Can you work these out from the model? Positions are in its coordinate system, mm. Face numbers are marked on the shaded views. A direction names the side the tool comes from. Give positions to 0.01 mm unless a question says otherwise; leave off trailing zeros. Order: outer loops, then holes, each group sorted by start corner. A loop starts at its lowest first (then second) coordinate and runs counter-clockwise, first axis right, second up. Notation, with made-up numbers: M -26.5,-15 L 9.5,-15 A21 cw 9.5,-1 Z; hole C -26.75,40 d6. An arc over 180 degrees is marked long. Answer as a JSON object with one key per item and string values.
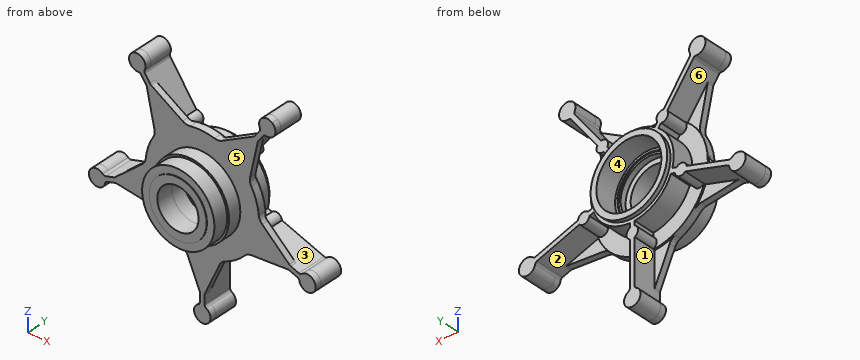
```python
from build123d import *
from build123d.topology import SkipClean

# Parameters (mm, degrees)
BOSS_EXTRUDE1_DEPTH     = 21
CIRPATTERN1_COUNT       = 5
SKETCH3_R               = 294.674158119
SKETCH3_R_2             = 133.5
CUT_EXTRUDE1_DEPTH      = 3.5
BOSS_EXTRUDE2_START     = 68
BOSS_EXTRUDE2_DEPTH     = 68
CIRPATTERN2_COUNT       = 5
SKETCH6_R               = 312.065811201
CUT_EXTRUDE3_DEPTH      = 15
SKETCH7_R               = 90
SKETCH7_R_2             = 71
BOSS_EXTRUDE3_DEPTH     = 9
SKETCH8_R               = 76.5
CUT_EXTRUDE4_DEPTH      = 50
SKETCH9_R               = 313.84536257
SKETCH9_R_2             = 94
CUT_EXTRUDE5_DEPTH      = 3
SKETCH10_R              = 106.760596323
SKETCH10_R_2            = 85
CUT_EXTRUDE6_DEPTH      = 34
SKETCH11_R              = 112.872926099
SKETCH11_R_2            = 89.5
CUT_EXTRUDE7_DEPTH      = 30
SKETCH12_R              = 67.5
SKETCH12_R_2            = 45
BOSS_EXTRUDE4_DEPTH     = 1
CUT_EXTRUDE8_DEPTH      = 412.038532061
CUT_EXTRUDE8_DEPTH_BACK = 412.038532061
SKETCH13_R              = 48.5


with BuildPart() as part:
    # Sketch1 → Revolve1 (revolve)
    with BuildSketch(Plane.XY, mode=Mode.PRIVATE) as revolve1_sk:
        with BuildLine():
            Line((89.84228169, 2.60989789), (97.5, 61))
            Line((97.5, 61), (133.5, 61))
            Line((133.5, 61), (133.5, 82))
            Line((133.5, 82), (97.5, 82))
            Line((97.5, 82), (97.5, 147))
            Line((97.5, 147), (71, 147))
            Line((71, 147), (71, 88))
            Line((71, 88), (66, 88))
            Line((66, 88), (66, 75))
            Line((66, 75), (54, 75))
            Line((54, 75), (51.505319297, 40.981626783))
            Line((51.505319297, 40.981626783), (50.883331755, 40.539778313))
            Line((50.883331755, 40.539778313), (48.5, 0))
            Line((48.5, 0), (86.867753099, 0))
            ThreePointArc((86.867753099, 0), (88.846350287, 0.744971582), (89.84228169, 2.60989789))
        make_face()
    revolve(revolve1_sk.sketch.rotate(Axis((0, 165, 0), (0, -1, 0)), 180), axis=Axis((0, 165, 0), (0, -1, 0)))

    # Sketch2 → Boss-Extrude1 (add)
    with BuildSketch(Plane(origin=(0, 82, 0), x_dir=(1, 0, 0), z_dir=(0, 1, 0))):
        with BuildLine():
            Line((-6.35450353, 213.067894216), (-40.878618186, 135.005909342))
            ThreePointArc((-40.878618186, 135.005909342), (-46.087052335, 127.41774711), (-53.688359463, 122.228515733))
            ThreePointArc((-53.688359463, 122.228515733), (0, 133.5), (53.688359463, 122.228515733))
            ThreePointArc((53.688359463, 122.228515733), (46.087052335, 127.41774711), (40.878618186, 135.005909342))
            Line((40.878618186, 135.005909342), (6.35450353, 213.067894216))
            ThreePointArc((6.35450353, 213.067894216), (5.71595777, 215.045623904), (5.5, 217.112630835))
            Line((5.5, 217.112630835), (5.5, 236.859260412))
            ThreePointArc((5.5, 236.859260412), (6.48800918, 240.444782185), (9.173133251, 243.018152978))
            ThreePointArc((9.173133251, 243.018152978), (18.712249031, 264.730881325), (0, 279.301023339))
            ThreePointArc((0, 279.301023339), (-18.712249031, 264.730881325), (-9.173133251, 243.018152978))
            ThreePointArc((-9.173133251, 243.018152978), (-6.48800918, 240.444782185), (-5.5, 236.859260412))
            Line((-5.5, 236.859260412), (-5.5, 217.112630835))
            ThreePointArc((-5.5, 217.112630835), (-5.71595777, 215.045623904), (-6.35450353, 213.067894216))
        make_face()
    boss_extrude1 = extrude(amount=-BOSS_EXTRUDE1_DEPTH)

    # CirPattern1: Boss-Extrude1 ×5 about axis
    cirpattern1_axis = Axis((0, 0, 0), (0, 1, 0))
    for i in range(1, CIRPATTERN1_COUNT):
        add(boss_extrude1.rotate(cirpattern1_axis, i * 360 / CIRPATTERN1_COUNT))

    # Sketch3 → Cut-Extrude1 (cut)
    with BuildSketch(Plane(origin=(0, 82, 0), x_dir=(1, 0, 0), z_dir=(0, 1, 0))):
        Circle(SKETCH3_R)
        with Locations(Location((0, 0, 0), (0, 0, 180))):
            Circle(SKETCH3_R_2, mode=Mode.SUBTRACT)
    extrude(amount=-CUT_EXTRUDE1_DEPTH, mode=Mode.SUBTRACT)

    # Sketch4 → Boss-Extrude2 (add)
    with SkipClean():  # the faces are left unmerged after this step: merging them gives an invalid solid
        with BuildSketch(Plane(origin=(0, 78.5, 0), x_dir=(1, 0, 0), z_dir=(0, 1, 0)).offset(BOSS_EXTRUDE2_START)):
            with BuildLine():
                Line((-5.5, 236.859260412), (-5.5, 132.328828006))
                ThreePointArc((-5.5, 132.328828006), (-13.5, 120), (-5.5, 107.671171994))
                Line((-5.5, 107.671171994), (-5.5, 97.344748189))
                ThreePointArc((-5.5, 97.344748189), (0, 97.5), (5.5, 97.344748189))
                Line((5.5, 97.344748189), (5.5, 107.671171994))
                ThreePointArc((5.5, 107.671171994), (13.5, 120), (5.5, 132.328828006))
                Line((5.5, 132.328828006), (5.5, 236.859260412))
                ThreePointArc((5.5, 236.859260412), (6.48800918, 240.444782185), (9.173133251, 243.018152978))
                ThreePointArc((9.173133251, 243.018152978), (0, 279.301023339), (-9.173133251, 243.018152978))
                ThreePointArc((-9.173133251, 243.018152978), (-6.48800918, 240.444782185), (-5.5, 236.859260412))
            make_face()
        boss_extrude2 = extrude(amount=-BOSS_EXTRUDE2_DEPTH)
    add(part.part.scale(1), mode=Mode.REPLACE)  # the faces are merged on a copy

    # CirPattern2: Boss-Extrude2 ×5 about axis
    cirpattern2_axis = Axis((0, 0, 0), (0, 1, 0))
    for i in range(1, CIRPATTERN2_COUNT):
        add(boss_extrude2.rotate(cirpattern2_axis, i * 360 / CIRPATTERN2_COUNT))

    # Sketch6 → Cut-Extrude3 (cut)
    with BuildSketch(Plane(origin=(0, 147, 0), x_dir=(1, 0, 0), z_dir=(0, 1, 0))):
        Circle(SKETCH6_R)
    extrude(amount=-CUT_EXTRUDE3_DEPTH, mode=Mode.SUBTRACT)

    # Sketch7 → Boss-Extrude3 (add)
    with BuildSketch(Plane(origin=(0, 132, 0), x_dir=(1, 0, 0), z_dir=(0, 1, 0))):
        with Locations(Location((0, 0, 0), (0, 0, 180))):
            Circle(SKETCH7_R)
        with Locations(Location((0, 0, 0), (0, 0, 180))):
            Circle(SKETCH7_R_2, mode=Mode.SUBTRACT)
    extrude(amount=BOSS_EXTRUDE3_DEPTH)

    # Sketch8 → Cut-Extrude4 (cut)
    with BuildSketch(Plane(origin=(0, 141, 0), x_dir=(1, 0, 0), z_dir=(0, 1, 0))):
        with Locations(Location((0, 0, 0), (0, 0, 180))):
            Circle(SKETCH8_R)
    extrude(amount=-CUT_EXTRUDE4_DEPTH, mode=Mode.SUBTRACT)

    # Sketch9 → Cut-Extrude5 (cut)
    with BuildSketch(Plane.XZ.offset(-61)):
        Circle(SKETCH9_R)
        Circle(SKETCH9_R_2, mode=Mode.SUBTRACT)
    extrude(amount=-CUT_EXTRUDE5_DEPTH, mode=Mode.SUBTRACT)

    # Sketch10 → Cut-Extrude6 (cut)
    with BuildSketch(Plane.XZ):
        Circle(SKETCH10_R)
        Circle(SKETCH10_R_2, mode=Mode.SUBTRACT)
    extrude(amount=-CUT_EXTRUDE6_DEPTH, mode=Mode.SUBTRACT)

    # Sketch11 → Cut-Extrude7 (cut)
    with BuildSketch(Plane.XZ.offset(-34)):
        Circle(SKETCH11_R)
        Circle(SKETCH11_R_2, mode=Mode.SUBTRACT)
    extrude(amount=-CUT_EXTRUDE7_DEPTH, mode=Mode.SUBTRACT)

    # Sketch12 → Boss-Extrude4 (add)
    with BuildSketch(Plane.XZ):
        with Locations(Location((0, 0, 0), (0, 0, 180))):
            Circle(SKETCH12_R)
        Circle(SKETCH12_R_2, mode=Mode.SUBTRACT)
    extrude(amount=BOSS_EXTRUDE4_DEPTH)

    # Sketch13 → Cut-Extrude8 (cut, two sides: drawn at the far end of the back side and taken through both)
    with BuildSketch(Plane(origin=(0, 0, 0), x_dir=(1, 0, 0), z_dir=(0, 1, 0)).offset(-CUT_EXTRUDE8_DEPTH_BACK)):
        with Locations(Location((0, 0, 0), (0, 0, 180))):
            Circle(SKETCH13_R)
    extrude(amount=CUT_EXTRUDE8_DEPTH + CUT_EXTRUDE8_DEPTH_BACK, mode=Mode.SUBTRACT)


solid = part.part
```
1) I want a section at B-B on z = -164.5. Write out the boundary of the cut face in (x, y), and give its area (3 significant figures).
Results found:
{"outline": "M -27.83,64 L 27.83,64 L 27.83,78.5 L 5.5,78.5 L 5.5,132 L -5.5,132 L -5.5,78.5 L -27.83,78.5 Z", "area": "1,400 mm²"}
2) For the marked faces 1, 2 and 3, which set-ups out of +Z, -Z, +X, -X, +Y, -Y let a thin tool reach every point of the face, with its end or its side?
Results found:
{"face 1": "-X, +Y", "face 2": "-Z, +Y", "face 3": "+Y"}
3) I'm going to push flat-ended pins straight in: pin 1 Ø2 at (y, z) = (26, -54.5) entering from +X; pin 2 Ø15 at (x, z) = (96.5, 99.5) entering from +Y; pin 3 Ø6 at (x, z) = (21, -159) entering from -Y. Where does each tip first touch, or does it pass through?
Results found:
{"pin 1": "stops at x = 66.05", "pin 2": "stops at y = 82", "pin 3": "stops at y = 64"}
4) I want a section at A-A on y = 55.5. Write out the boundary of the cut face in (x, z).
Results found:
{"outline": "C 0,0 d179; hole C 0,0 d105.14"}
5) I need wall thicknesses on L1, parallel to Z at x = 0, y = 83.25; L2, parallel to Z at x = 69, y = 123; L3, parallel to Z at x = 0, y = -0.7. Which ranges of each line are inside material? Lowest first, please.
Results found:
{"L1": "z = -279.3 to -66, 66 to 97.5", "L2": "z = -68.89 to -33.03, 33.03 to 68.89, 83.67 to 110.49", "L3": "z = -67.5 to -48.5, 48.5 to 67.5"}
6) I want a section at C-C on y = 19. Write out the boundary of the cut face in (x, z), and give its area (3 significant figures).
Results found:
{"outline": "C 0,0 d170; hole C 0,0 d99.23", "area": "15,000 mm²"}
7) Thinking about a two-plate mould opening in X: for the marked faces 4, 5 and 6, which applies, pulls with the +X half, pulls with the -X half, needs draft (parallel to the pull), parting line crosses it, or undercut?
Results found:
{"face 4": "undercut", "face 5": "needs draft", "face 6": "pulls with the -X half"}
